from build123d import *

# Parameters (mm, degrees)
F1_ANGLE = 180
F2_R     = 3


with BuildPart() as f1:
    # F0 (on Front) → F1 (revolve)
    with BuildSketch(Plane.XZ):
        Polygon((-26.7573259016, 0.2080155462), (-15.7573259016, 0.2080155462), (-15.7573259016, 21.2080155462), (-21.2573259016, 21.2080155462), (-21.2573259016, 29.2080155462), (-0.0573259016, 29.2080155462), (-0.0573259016, 34.6219648462), (-26.7573259016, 34.6219648462), (-26.7573259016, 29.1219648462), (-26.7573259016, 23.8824076951), (-26.7573259016, 8.0824076951), align=None)
    revolve(axis=Axis((-0.0573259016, 0, 3.4359856569), (0, 0, 1)), revolution_arc=F1_ANGLE)

    # F2
    f2_edges = [f1.edges().sort_by_distance(p)[0] for p in [
        (-0.057326, -26.7, 34.621965),
    ]]
    fillet(f2_edges, radius=F2_R)


solid = f1.part
Work out the finished part from the listing and answer in its coordinate system (mm). A direction names the side the tool comes from. Round coordinates to 2 decimals unless told otherwise and drop trailing zeros. Write each loop counter-clockwise with the first axis right and the second up, starting at its lowest first coordinate (ties: lowest second). Pieces come first, ordered by that corner, then holes. Notation, with made-up numbers: (46.25, 25) - (98.25, 25) arc R19 ccw to (98.25, 41) - close; hole circle Ø1 at (-16.75, -0.5). An arc over 180 degrees is marked (long way). Answer in a Markdown table with one row per item. Add a question column.
1. A cutting plane is placed at A-A, the plane z = 26. Determine the outline of the cut face in (x, y), and give its area (3 significant figures).
2. The mould has two halves that part along Z. Classify faces 4 (the flat face through (0, -9, 34.622)), 5 (the flat face through (0, -17, 0.208)), 6 (the flat face through (0, -18, 21.208)), 7 (the flat face through (0, 0, 33)): +Z half, -Z half, draft (parallel to the pull), parting line (faces both ways), or undercut.
3. Given pin 1 (6 mm diameter, centred on y = -4, z = 26.5, fed in from -X); pin 2 (8 mm diameter, centred on y = -12, z = 30, fed in from -X); pin 3 (1 mm diameter, centred on x = 1, z = 11.5, fed in from -Y), each flat-ended and moving along its own axis, determine where each tip first touches the part or whether it passes through.
4. A cutting plane is placed at B-B, the plane z = 11. Determine the outline of the cut face in (x, y).
5. Find the intervals of material crossed by line 1 along Z through (x, y) = (0.5, -16); line 2 along X through (y, z) = (-12.5, 4); line 3 along Y through (x, z) = (-0.5, 30), in increasing order. Write a range as from..to.
6. For faces 1 (the cylindrical face through (-0.644, -26.694, 15.695)), 2 (the cylindrical face through (-0.403, -15.696, 10.855)), 3 (the cylindrical face through (-0.524, -21.195, 25.264)), determine the directions among +Z, -Z, +X, -X, +Y, -Y from which every point of the face is accessible in a straight line to the end or side of a thin tool.
Worked out:
| question | item | result |
|---|---|---|
| 1 | outline | (-26.76, 0) arc R26.7 ccw to (26.64, 0) - (21.14, 0) arc R21.2 cw to (-21.26, 0) - close |
| 1 | area | 414 mm^2 |
| 2 | face 4 | +Z half |
| 2 | face 5 | -Z half |
| 2 | face 6 | undercut |
| 2 | face 7 | draft |
| 3 | pin 1 | x = -26.74 |
| 3 | pin 2 | x = -25.53 |
| 3 | pin 3 | y = -26.69 |
| 4 | outline | (-26.76, 0) arc R26.7 ccw to (26.64, 0) - (15.64, 0) arc R15.7 cw to (-15.76, 0) - close |
| 5 | line 1 | 0.21..21.21, 29.21..34.62 |
| 5 | line 2 | -23.65..-9.56, 9.44..23.54 |
| 5 | line 3 | -26.7..0 |
| 6 | face 1 | +Z, -Z, -Y |
| 6 | face 2 | -Z, +Y |
| 6 | face 3 | +Y |
